The listing builds one solid part. Answer for the finished solid, in the listing's coordinates (mm). Face numbers are marked on the shaded views. A direction names the side the tool comes from. Coordinates: 2 decimals unless noted, no trailing zeros. Order: outer loops, then holes, each group sorted by start corner. A loop starts at its lowest first (then second) coordinate and runs counter-clockwise, first axis right, second up. Notation, with made-up numbers: (21.5, -19) - (67.5, -19) arc R32 cw to (67.5, 19) - close; hole circle Ø2 at (-4.75, -7.75). An arc over 180 degrees is marked (long way). Use a Markdown table: item, result. Add a question column.
Item 1: The part is cut by section A-A, the plane x = 25. Give the vertices of the cut face in (y, z).
Item 2: Flat-ended cylindrical pins translate along their axes: P1, Ø4, axis at y = 13, z = 6, coming from the -X side; P2, Ø6, axis at x = 56, y = 6.5, coming from the +Z side; P3, Ø4, axis at x = -50, z = 7, coming from the -Y side; P4, Ø4, axis at x = 104, z = 7, coming from the +Y side. Find the tip coordinate at first contact, or state that the pin passes through.
Item 3: The part is cut by section B-B, the plane y = 11. State how many separate pieces and enclosed holes the cut face has, then the cut area to 3 significant figures.
Item 4: For the marked faces 1 and 2, determine the directions among +Z, -Z, +X, -X, +Y, -Y from which every point of the face is accessible in a straight line to the end or side of a thin tool.
Item 5: The part is cut by section C-C, the plane x = -31. Give the vertices of the cut face in (y, z).
Item 6: The mould has two halves that part along X. Classify the marked faces 3 and 4: released by +X, released by -X, zero draft, split by the parting line, or undercut.
Item 7: Find the intervals of material crossed by line 1 along Z through (x, y) = (145, 1.6); line 2 along X through (y, z) = (16.5, 2.75); line 3 along Y through (x, z) = (-3.5, 7), in increasing order.
from build123d import *

# Parameters (mm, degrees)
EXTRU_MINCE1_DEPTH           = 14
CONG_1_R                     = 2
CONG_2_R                     = 1
CONG_3_R                     = 2
ENL_V_MAT_EXTRU_1_DEPTH      = 151.73486657
ENL_V_MAT_EXTRU_1_DEPTH_BACK = 151.73486657
ESQUISSE2_R                  = 1.75
CHANFREIN1_SIZE              = 1.3


with BuildPart() as part:
    # Esquisse1 → Extru.-Mince1 (new body)
    with BuildSketch(Plane.XY):
        with BuildLine():
            Line((-149, 0), (-133.660254038, 0))
            ThreePointArc((-133.660254038, 0), (-125, 15), (-116.339745962, 0))
            Line((-116.339745962, 0), (-83.660254038, 0))
            ThreePointArc((-83.660254038, 0), (-75, 15), (-66.339745962, 0))
            Line((-66.339745962, 0), (-33.660254038, 0))
            ThreePointArc((-33.660254038, 0), (-25, 15), (-16.339745962, 0))
            Line((-16.339745962, 0), (16.339745962, 0))
            ThreePointArc((16.339745962, 0), (25, 15), (33.660254038, 0))
            Line((33.660254038, 0), (66.339745962, 0))
            ThreePointArc((66.339745962, 0), (75, 15), (83.660254038, 0))
            Line((83.660254038, 0), (116.339745962, 0))
            ThreePointArc((116.339745962, 0), (125, 15), (133.660254038, 0))
            Line((133.660254038, 0), (149, 0))
            Line((149, 0), (149, 3))
            Line((149, 3), (137.845232579, 3))
            ThreePointArc((137.845232579, 3), (125, 18), (112.154767421, 3))
            Line((112.154767421, 3), (87.845232579, 3))
            ThreePointArc((87.845232579, 3), (75, 18), (62.154767421, 3))
            Line((62.154767421, 3), (37.845232579, 3))
            ThreePointArc((37.845232579, 3), (25, 18), (12.154767421, 3))
            Line((12.154767421, 3), (-12.154767421, 3))
            ThreePointArc((-12.154767421, 3), (-25, 18), (-37.845232579, 3))
            Line((-37.845232579, 3), (-62.154767421, 3))
            ThreePointArc((-62.154767421, 3), (-75, 18), (-87.845232579, 3))
            Line((-87.845232579, 3), (-112.154767421, 3))
            ThreePointArc((-112.154767421, 3), (-125, 18), (-137.845232579, 3))
            Line((-137.845232579, 3), (-149, 3))
            Line((-149, 3), (-149, 0))
        make_face()
    extrude(amount=EXTRU_MINCE1_DEPTH)

    # Congé1
    cong_1_edges = [part.edges().sort_by_distance(p)[0] for p in [
        (133.660254038, 0, 7),
        (116.339745962, 0, 7),
        (83.660254038, 0, 7),
        (66.339745962, 0, 7),
        (33.660254038, 0, 7),
        (16.339745962, 0, 7),
        (-16.339745962, 0, 7),
        (-33.660254038, 0, 7),
        (-66.339745962, 0, 7),
        (-83.660254038, 0, 7),
        (-116.339745962, 0, 7),
        (-133.660254038, 0, 7),
    ]]
    fillet(cong_1_edges, radius=CONG_1_R)

    # Congé2
    cong_2_edges = [part.edges().sort_by_distance(p)[0] for p in [
        (-137.845232579, 3, 7),
        (-112.154767421, 3, 7),
        (-87.845232579, 3, 7),
        (-62.154767421, 3, 7),
        (-37.845232579, 3, 7),
        (-12.154767421, 3, 7),
        (12.154767421, 3, 7),
        (37.845232579, 3, 7),
        (62.154767421, 3, 7),
        (87.845232579, 3, 7),
        (112.154767421, 3, 7),
        (137.845232579, 3, 7),
    ]]
    fillet(cong_2_edges, radius=CONG_2_R)

    # Congé3
    cong_3_edges = [part.edges().sort_by_distance(p)[0] for p in [
        (149, 3, 7),
        (-149, 3, 7),
    ]]
    fillet(cong_3_edges, radius=CONG_3_R)

    # Esquisse2 → Enlèv. mat.-Extru.1 (cut, two sides: drawn at the far end of the back side and taken through both)
    with BuildSketch(Plane.XZ.offset(-ENL_V_MAT_EXTRU_1_DEPTH_BACK)):
        with Locations((-145, 7)):
            Circle(ESQUISSE2_R)
        with Locations((145, 7)):
            Circle(ESQUISSE2_R)
        with Locations(Location((-50, 7, 0), (0, 0, 270))):
            Circle(ESQUISSE2_R)
        with Locations(Location((50, 7, 0), (0, 0, 270))):
            Circle(ESQUISSE2_R)
    extrude(amount=ENL_V_MAT_EXTRU_1_DEPTH + ENL_V_MAT_EXTRU_1_DEPTH_BACK, mode=Mode.SUBTRACT)

    # Chanfrein1
    chanfrein1_edges = [part.edges().sort_by_distance(p)[0] for p in [
        (-146.75, 0, 7),
        (50, 0, 8.75),
        (-50, 0, 8.75),
        (143.25, 0, 7),
    ]]
    chamfer(chanfrein1_edges, length=CHANFREIN1_SIZE)


solid = part.part
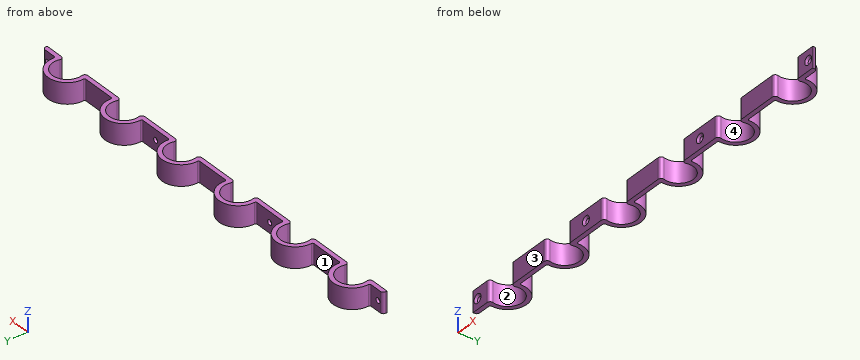
Solution:
| question | item | result |
|---|---|---|
| 1 | outline | (15, 0) - (18, 0) - (18, 14) - (15, 14) - close |
| 2 | P1 | stops at x = -136.53 |
| 2 | P2 | passes through |
| 2 | P3 | stops at y = 1.05 |
| 2 | P4 | stops at y = 3 |
| 3 | separate pieces | 12 |
| 3 | enclosed holes | 0 |
| 3 | area | 593 mm2 |
| 4 | face 1 | +Z, -Z, +Y |
| 4 | face 2 | +Z, -Z |
| 5 | outline | (13, 0) - (16.53, 0) - (16.53, 14) - (13, 14) - close |
| 6 | face 3 | zero draft |
| 6 | face 4 | undercut |
| 7 | line 1 | z = 0 to 5.25, 8.75 to 14 |
| 7 | line 2 | x = -131.06 to -118.94, -81.06 to -68.94, -31.06 to -18.94, 18.94 to 31.06, 68.94 to 81.06, 118.94 to 131.06 |
| 7 | line 3 | y = 0 to 3 |
